Here's how the part is built. I have some questions about the finished solid (model axes, mm). Round coordinates to 2 decimals unless told otherwise and drop trailing zeros. Write each loop counter-clockwise with the first axis right and the second up, starting at its lowest first coordinate (ties: lowest second). Pieces come first, ordered by that corner, then holes. Notation, with made-up numbers: (56, -35) -> (108, -35) arc R20 ccw to (108, -7) -> close; hole circle Ø8 at (-11.5, 84). An arc over 180 degrees is marked (long way). Put each result on its own line as item: value. Start each with the question number.
1) If I drill on line 1 along Y through (x, z) = (80.5, 2.45); line 2 along Y through (x, z) = (42.5, 0.95); line 3 along X through (y, z) = (59, 2.6), over which ranges is the centre line in solid material (lowest first)? Write a range as [from, to].
2) I want a section at B-B, the plane y = 75.5. List the corners of the cut face in (x, z) for me, then the cut area to 3 significant figures.
3) I want a section at A-A, the plane z = 1.5. List the corners of the cut face in (x, y) for me.
4) I want a section at C-C, the plane x = 8. List the corners of the cut face in (y, z) for me.
from build123d import *

# Parameters (mm, degrees)
BASE_EXTRUDE_DEPTH = 5


with BuildPart() as part:
    # Sketch2 → Base-Extrude (new body)
    with BuildSketch(Plane.XY):
        with BuildLine():
            Line((48.116224765, 92), (-5, 0))
            Line((-5, 0), (83.61203206, 0))
            ThreePointArc((83.61203206, 0), (103.33761172, 8.563582044), (110.550478804, 28.822110589))
            Line((110.550478804, 28.822110589), (107.902603037, 67.968834584))
            ThreePointArc((107.902603037, 67.968834584), (105.920101953, 74.468797721), (101.27285986, 79.426919569))
            Line((101.27285986, 79.426919569), (86.248315424, 89.470368646))
            ThreePointArc((86.248315424, 89.470368646), (82.267967787, 91.353667296), (77.912254854, 92))
            Line((77.912254854, 92), (48.116224765, 92))
        make_face()
    extrude(amount=BASE_EXTRUDE_DEPTH)


solid = part.part
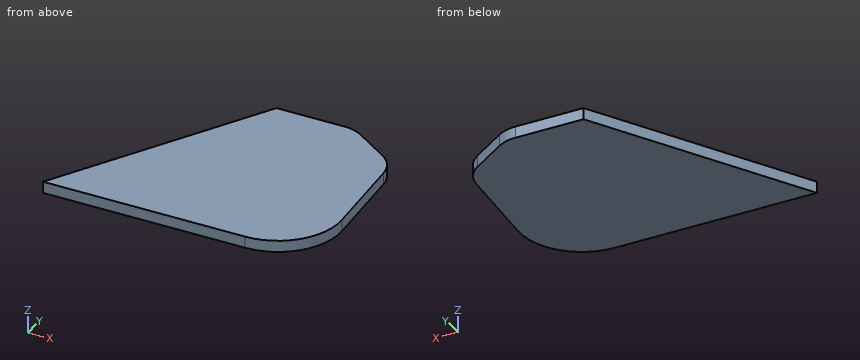
Findings:
1. line 1: y = [0, 91.78]
1. line 2: y = [0, 82.27]
1. line 3: x = [29.06, 108.51]
2. outline: (38.59, 0) -> (105.27, 0) -> (105.27, 5) -> (38.59, 5) -> close
2. area: 333 mm2
3. outline: (-5, 0) -> (83.61, 0) arc R27 ccw to (110.55, 28.82) -> (107.9, 67.97) arc R15 ccw to (101.27, 79.43) -> (86.25, 89.47) arc R15 ccw to (77.91, 92) -> (48.12, 92) -> close
4. outline: (0, 0) -> (22.52, 0) -> (22.52, 5) -> (0, 5) -> close
